For this review, use the dimensioned drawing (mm, ordinates from the lowest corner) and the shaded views. A direction names the side the tool comes from. Round coordinates to 2 decimals unless told otherwise and drop trailing zeros. Loops run counter-clockwise (first coordinate to the right, second up) from the corner with the lowest first, then second, coordinate; pieces in that order, holes last. Notation, with made-up numbers: (2, -0.75) -> (40, -0.75) arc R26 cw to (40, 17.25) -> close; hole circle Ø4 at (-35.5, 23). An arc over 180 degrees is marked (long way). Write each question's results on one line, items separated by ' | '.
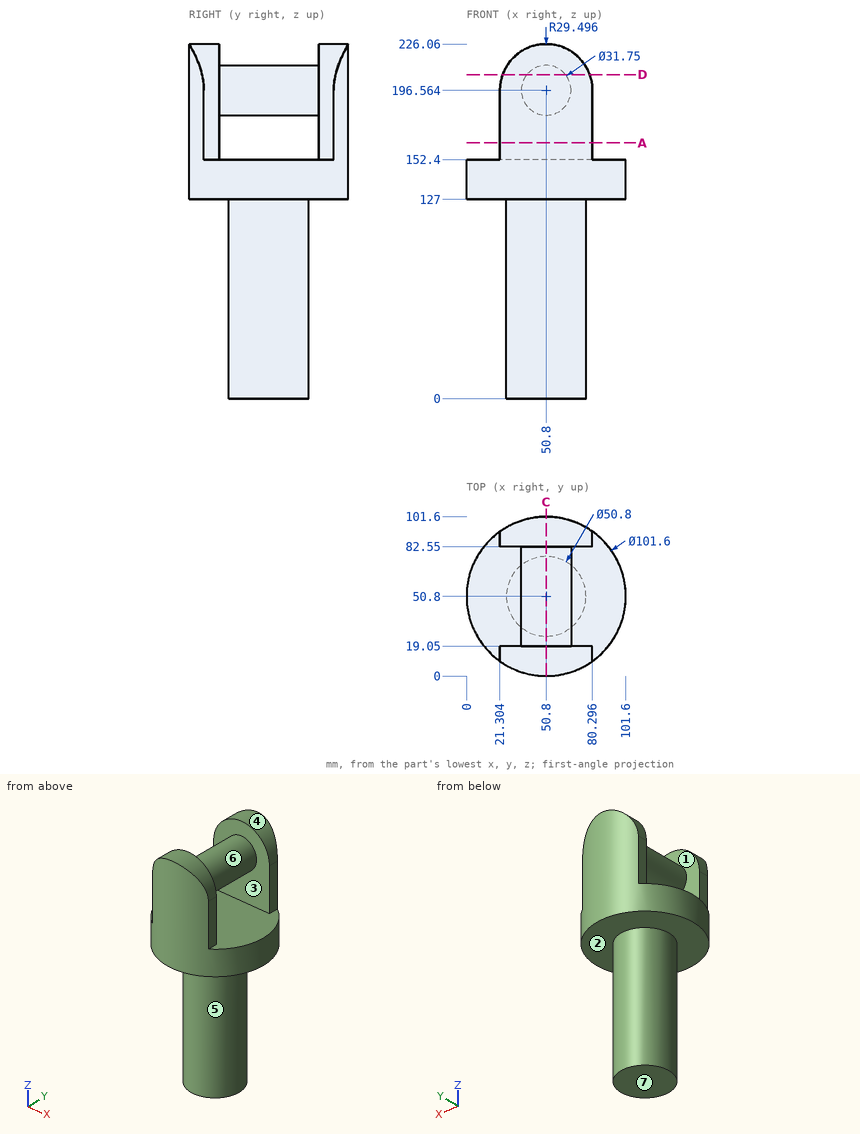
1. Draft analysis for pull direction Z (two halves, no side actions). For the marked faces 1, 2, 3 and 4, state which applies: released by +Z, released by -Z, zero draft, split by the parting line, or undercut.
Values found:
face 1: undercut | face 2: released by -Z | face 3: undercut | face 4: released by +Z
2. For pin 1 (5 mm diameter, centred on y = 16, z = 165.5, fed in from -X); pin 2 (4 mm diameter, centred on x = 32.5, z = 131.5, fed in from -Y); pin 3 (10 mm diameter, centred on y = 69, z = 45, fed in from -X), all flat-tipped, find the tip position at first contact; note any pin that passes through.
Values found:
pin 1: stops at x = 21.3 | pin 2: stops at y = 2.69 | pin 3: stops at x = 29.1
3. Consider section D-D (z = 206.5). State the section outline as (x, y) points.
Values found:
outline: (23.03, 8.26) arc R50.8 ccw to (78.57, 8.26) -> (78.57, 19.05) -> (63.18, 19.05) -> (63.18, 82.55) -> (78.57, 82.55) -> (78.57, 93.34) arc R50.8 ccw to (23.03, 93.34) -> (23.03, 82.55) -> (38.42, 82.55) -> (38.42, 19.05) -> (23.03, 19.05) -> close
4. Consider section C-C (x = 50.8). State the section outline as (y, z) points.
Values found:
outline: (0, 127) -> (25.4, 127) -> (25.4, 0) -> (76.2, 0) -> (76.2, 127) -> (101.6, 127) -> (101.6, 226.06) -> (82.55, 226.06) -> (82.55, 212.44) -> (19.05, 212.44) -> (19.05, 226.06) -> (0, 226.06) -> close; hole (19.05, 152.4) -> (82.55, 152.4) -> (82.55, 180.69) -> (19.05, 180.69) -> close
5. Tool access review of the marked faces 5, 6 and 7: name each direction out of +Z, -Z, +X, -X, +Y, -Y from which nothing blocks a thin tool from reaching the whole face with its end or side.
Values found:
face 5: -Z | face 6: none | face 7: -Z, +X, -X, +Y, -Y
6. To check wall thickness, follow probe 1 along Z at (x, y) = (25, 59.5); probe 2 along X at (y, z) = (27.5, 195.5); probe 3 along Z at (x, y) = (49, 50). State the ranges of each line that lie inside material, in increasing order.
Values found:
probe 1: z = 127 to 152.4 | probe 2: x = 34.96 to 66.64 | probe 3: z = 0 to 152.4, 180.79 to 212.34
7. Consider section A-A (z = 163). State the section outline as (x, y) points.
Values found:
outline: (21.3, 9.44) arc R50.8 ccw to (80.3, 9.44) -> (80.3, 19.05) -> (21.3, 19.05) -> close; (21.3, 82.55) -> (80.3, 82.55) -> (80.3, 92.16) arc R50.8 ccw to (21.3, 92.16) -> close
